The listing builds one solid part. Answer for the finished solid, in the listing's coordinates (mm). Face numbers are marked on the shaded views. Round coordinates to 2 decimals unless told otherwise and drop trailing zeros. Write each loop counter-clockwise with the first axis right and the second up, starting at its lowest first coordinate (ties: lowest second). Pieces come first, ordered by that corner, then holes. Notation, with made-up numbers: M 2,46.25 L 18,46.25 A19 cw 18,72.25 Z; hole C -30.5,-31.75 d1. An arc over 180 degrees is marked long. Put each result on its own line as item: value. Start each with the question number.
```python
from build123d import *

# Parameters (mm, degrees)
F0_R     = 16.05
F0_R_2   = 14.85
F0_R_3   = 1.5
F1_DEPTH = 2
F2_DEPTH = 3.65
F3_SIZE  = 1.5


with BuildPart() as f1:
    # F0 (on Top) → F1 (new body)
    with BuildSketch(Plane.XY):
        Circle(F0_R)
        Circle(F0_R_2, mode=Mode.SUBTRACT)
        Circle(F0_R_2)
        Circle(F0_R_3, mode=Mode.SUBTRACT)
    extrude(amount=-F1_DEPTH)

    # F0 (on Top) → F2 (join)
    with BuildSketch(Plane.XY):
        Circle(F0_R)
        Circle(F0_R_2, mode=Mode.SUBTRACT)
    extrude(amount=F2_DEPTH)

    # F3
    f3_edges = [f1.edges().sort_by_distance(p)[0] for p in [
        (-1.5, 0, 0),
    ]]
    chamfer(f3_edges, length=F3_SIZE)


solid = f1.part
```
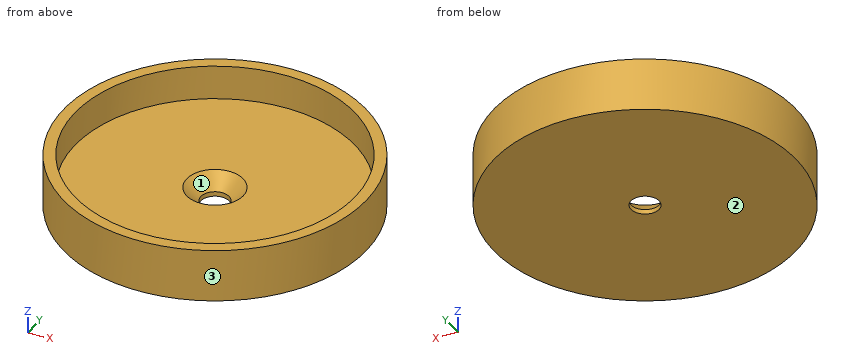
Item 1: Flat-ended cylindrical pins translate along their axes: pin 1 (15 mm diameter, centred on x = -2, y = -1, fed in from +Z); pin 2 (2 mm diameter, centred on x = 5, z = 0, fed in from -Y). Find the tip coordinate at first contact, or state that the pin passes through.
Item 2: Section A-A (x = 0) is taken. Give the vertices of the cut face in (y, z), and give its area (3 significant figures).
Item 3: Section C-C (z = 2.25) is taken. Give the vertices of the cut face in (x, y).
Item 4: Section D-D (y = -3.5) is taken. Give the vertices of the cut face in (x, z).
Item 5: Determine the mould class of the marked faces 1, 2 and 3 for opening direction Y: released by +Y, released by -Y, zero draft, split by the parting line, or undercut.
Item 6: Consider line 1 along Y through (x, z) = (0, -1.65); line 2 along Y through (x, z) = (0, 2.65); line 3 along Z through (x, y) = (-9, 10). Determine where each line is inside the solid, lowest interval first. Write a range as [from, to].
Output values:
1. pin 1: stops at z = 0
1. pin 2: stops at y = -15.54
2. outline: M -16.05,-2 L -1.5,-2 L -1.5,-1.5 L -3,0 L -14.85,0 L -14.85,3.65 L -16.05,3.65 Z; M 1.5,-2 L 16.05,-2 L 16.05,3.65 L 14.85,3.65 L 14.85,0 L 3,0 L 1.5,-1.5 Z
2. area: 64.7 mm^2
3. outline: C 0,0 d32.1; hole C 0,0 d29.7
4. outline: M -15.66,-2 L 15.66,-2 L 15.66,3.65 L 14.43,3.65 L 14.43,0 L -14.43,0 L -14.43,3.65 L -15.66,3.65 Z
5. face 1: undercut
5. face 2: zero draft
5. face 3: split by the parting line
6. line 1: y = [-16.05, -1.5], [1.5, 16.05]
6. line 2: y = [-16.05, -14.85], [14.85, 16.05]
6. line 3: z = [-2, 0]
